Can you work these out from the model? Positions are in its coordinate system, mm. Face numbers are marked on the shaded views. Give positions to 0.01 mm unless a question says otherwise; leave off trailing zeros. Order: outer loops, then holes, each group sorted by start corner. A loop starts at its lowest first (then second) coordinate and runs counter-clockwise, first axis right, second up. Notation, with made-up numbers: (45, -4) - (97, -4) arc R21 cw to (97, 25) - close; hole circle Ø7 at (24, 50.25). An arc over 180 degrees is marked (long way). Answer as CSV lines item,"result".
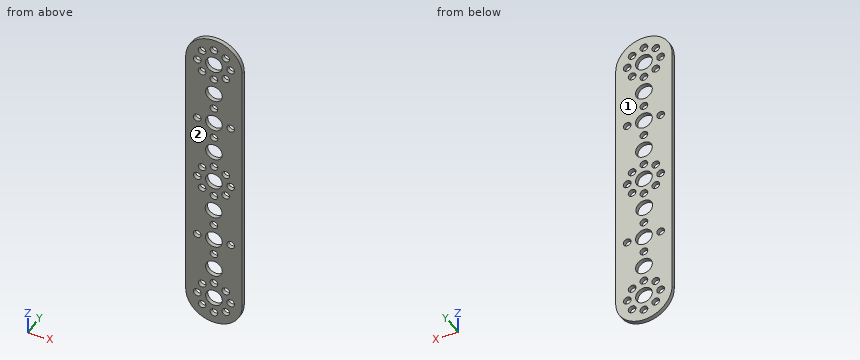
```python
from build123d import *

# Parameters (mm, degrees)
EXTRUDE1_DEPTH = 2
SKETCH2_R      = 4
SKETCH2_R_2    = 1.85
EXTRUDE2_DEPTH = 2


with BuildPart() as part:
    # Sketch1 → Extrude1 (new body)
    with BuildSketch(Plane(origin=(0, 0, 0), x_dir=(1, 0, 0), z_dir=(0, 1, 0))):
        with BuildLine():
            Line((-13.5, 64), (-13.5, -64))
            ThreePointArc((-13.5, -64), (0, -77.5), (13.5, -64))
            Line((13.5, -64), (13.5, 64))
            ThreePointArc((13.5, 64), (0, 77.5), (-13.5, 64))
        make_face()
    extrude(amount=EXTRUDE1_DEPTH)

    # Sketch2 → Extrude2 (cut)
    with BuildSketch(Plane(origin=(0, 2, 0), x_dir=(1, 0, 0), z_dir=(0, 1, 0))):
        with Locations((0, -48)):
            Circle(SKETCH2_R)
        with Locations((0, -16)):
            Circle(SKETCH2_R)
        with Locations((-0.175415159, 16)):
            Circle(SKETCH2_R)
        with Locations((0, 48)):
            Circle(SKETCH2_R)
        with Locations((0, -32)):
            Circle(SKETCH2_R)
        with Locations((0, -24)):
            Circle(SKETCH2_R_2)
        with Locations((0, -40)):
            Circle(SKETCH2_R_2)
        with Locations((8, -32)):
            Circle(SKETCH2_R_2)
        with Locations((-8, -32)):
            Circle(SKETCH2_R_2)
        with Locations((0, -56)):
            Circle(SKETCH2_R_2)
        with Locations((8, -64)):
            Circle(SKETCH2_R_2)
        with Locations((0, -64)):
            Circle(SKETCH2_R)
        with Locations((-8, -64)):
            Circle(SKETCH2_R_2)
        with Locations((-5.66, -69.66)):
            Circle(SKETCH2_R_2)
        with Locations((5.66, -69.66)):
            Circle(SKETCH2_R_2)
        with Locations((0, -72)):
            Circle(SKETCH2_R_2)
        with Locations((-5.66, -58.34)):
            Circle(SKETCH2_R_2)
        with Locations((5.66, -58.34)):
            Circle(SKETCH2_R_2)
        with Locations((0, 32)):
            Circle(SKETCH2_R)
        with Locations((0, 40)):
            Circle(SKETCH2_R_2)
        with Locations((0, 24)):
            Circle(SKETCH2_R_2)
        with Locations((8, 32)):
            Circle(SKETCH2_R_2)
        with Locations((-8, 32)):
            Circle(SKETCH2_R_2)
        with Locations((0, 8)):
            Circle(SKETCH2_R_2)
        with Locations((8, 0)):
            Circle(SKETCH2_R_2)
        Circle(SKETCH2_R)
        with Locations((-8, 0)):
            Circle(SKETCH2_R_2)
        with Locations((-5.66, -5.66)):
            Circle(SKETCH2_R_2)
        with Locations((5.66, -5.66)):
            Circle(SKETCH2_R_2)
        with Locations((0, -8)):
            Circle(SKETCH2_R_2)
        with Locations((-5.66, 5.66)):
            Circle(SKETCH2_R_2)
        with Locations((5.66, 5.66)):
            Circle(SKETCH2_R_2)
        with Locations((0, 56)):
            Circle(SKETCH2_R_2)
        with Locations((-8, 64)):
            Circle(SKETCH2_R_2)
        with Locations((0, 64)):
            Circle(SKETCH2_R)
        with Locations((8, 64)):
            Circle(SKETCH2_R_2)
        with Locations((5.66, 69.66)):
            Circle(SKETCH2_R_2)
        with Locations((-5.66, 69.66)):
            Circle(SKETCH2_R_2)
        with Locations((0, 72)):
            Circle(SKETCH2_R_2)
        with Locations((5.66, 58.34)):
            Circle(SKETCH2_R_2)
        with Locations((-5.66, 58.34)):
            Circle(SKETCH2_R_2)
    extrude(amount=-EXTRUDE2_DEPTH, mode=Mode.SUBTRACT)


solid = part.part
```
1) I want a section at C-C on y = 0.5. Count the separate pieces of the cut face and the enclosed holes in it, plus the area to 3 significant figures.
Answer block:
separate pieces,"1"
enclosed holes,"41"
area,"3,230 mm2"
2) I need wall thicknesses on line 1 along X through (y, z) = (0.7, 5.66); line 2 along X through (y, z) = (1.4, -32); line 3 along X through (y, z) = (1.3, 24). Which ranges of each line are inside material? Lowest first, please. Write a range as [from, to].
Answer block:
line 1,"[-13.5, -7.51], [-3.81, 3.81], [7.51, 13.5]"
line 2,"[-13.5, -9.85], [-6.15, -4], [4, 6.15], [9.85, 13.5]"
line 3,"[-13.5, -1.85], [1.85, 13.5]"
3) If we mould it in two halves opening along Y, with no side actions, what happens to the marked faces 1 and 2? For each: +Y half, -Y half, draft (parallel to the pull), parting line (faces both ways), or undercut.
Answer block:
face 1,"+Y half"
face 2,"-Y half"
4) I want a section at B-B on z = 0. Write out the boundary of the cut face in (x, y), plus the area to 3 significant figures.
Answer block:
outline,"(-13.5, 0) - (-9.85, 0) - (-9.85, 2) - (-13.5, 2) - close; (-6.15, 0) - (-4, 0) - (-4, 2) - (-6.15, 2) - close; (4, 0) - (6.15, 0) - (6.15, 2) - (4, 2) - close; (9.85, 0) - (13.5, 0) - (13.5, 2) - (9.85, 2) - close"
area,"23.2 mm2"
5) I want a section at D-D on z = -40. Write out the boundary of the cut face in (x, y), plus the area to 3 significant figures.
Answer block:
outline,"(-13.5, 0) - (-1.85, 0) - (-1.85, 2) - (-13.5, 2) - close; (1.85, 0) - (13.5, 0) - (13.5, 2) - (1.85, 2) - close"
area,"46.6 mm2"
6) I want a section at A-A on z = -16. Write out the boundary of the cut face in (x, y), plus the area to 3 significant figures.
Answer block:
outline,"(-13.5, 0) - (-4.18, 0) - (-4.18, 2) - (-13.5, 2) - close; (3.82, 0) - (13.5, 0) - (13.5, 2) - (3.82, 2) - close"
area,"38.0 mm2"
